Autodesk Fusion 360 part; units mm, degrees
sketch "Sketch1" plane through (0, 0, 0) normal (0, 0, 1) x (1, 0, 0)
  line L0 (0, 0) -> (-12.1, 6.9859) construction
  line L1 (0, 0) -> (0, -13.9719) construction
  line L2 (0, 0) -> (12.1, 6.9859) construction
  line L3 (12.1, -20.9578) -> (24.2, -13.9719)
  line L4 (24.2, -13.9719) -> (24.2, 0)
  line L5 (24.2, 0) -> (12.1, 6.9859)
  line L6 (12.1, 6.9859) -> (0, 0)
  line L7 (0, 0) -> (0, -13.9719)
  line L8 (0, -13.9719) -> (12.1, -20.9578)
  line L9 (12.1, 6.9859) -> (12.1, 20.9578)
  line L10 (12.1, 20.9578) -> (0, 27.9438)
  line L11 (0, 27.9438) -> (-12.1, 20.9578)
  line L12 (-12.1, 20.9578) -> (-12.1, 6.9859)
  line L13 (-12.1, 6.9859) -> (0, 0)
  line L14 (0, 0) -> (12.1, 6.9859) construction
  line L15 (0, -13.9719) -> (0, 0) construction
  line L16 (0, 0) -> (-12.1, 6.9859)
  line L17 (-12.1, 6.9859) -> (-24.2, 0)
  line L18 (-24.2, 0) -> (-24.2, -13.9719)
  line L19 (-24.2, -13.9719) -> (-12.1, -20.9578)
  line L20 (-12.1, -20.9578) -> (0, -13.9719)
  point P0 (12.1, -6.9859)
  point P1 (0, 13.9719)
  point P2 (-12.1, -6.9859)
  dimension "d3" = 120
  dimension "d4" = 120
  dimension "d5" = 12.1
  dimension "d6" = 12.1
  dimension "d7" = 12.1
extrude "Extrude1" add sketch "Sketch1" along normal blind 3
sketch "Sketch2" plane through (0, 0, 3) normal (0, 0, 1) x (1, 0, 0)
  line L0 (-12.1, -20.9578) -> (0, -13.9719)
  line L1 (0, -13.9719) -> (12.1, -20.9578)
  line L2 (12.1, -20.9578) -> (24.2, -13.9719)
  line L3 (24.2, -13.9719) -> (24.2, 0)
  line L4 (24.2, 0) -> (12.1, 6.9859)
  line L5 (12.1, 6.9859) -> (12.1, 20.9578)
  line L6 (12.1, 20.9578) -> (0, 27.9438)
  line L7 (0, 27.9438) -> (-12.1, 20.9578)
  line L8 (-12.1, 20.9578) -> (-12.1, 6.9859)
  line L9 (-12.1, 6.9859) -> (-24.2, 0)
  line L10 (-24.2, 0) -> (-24.2, -13.9719)
  line L11 (-24.2, -13.9719) -> (-12.1, -20.9578)
  line L12 (15, 1.1) -> (-15, 1.1)
  line L13 (-15, 1.1) -> (-15, 3.1)
  line L14 (-15, 3.1) -> (15, 3.1)
  line L15 (15, 3.1) -> (15, 1.1)
  line L16 (15, -1.1) -> (-15, -1.1)
  line L17 (-15, -1.1) -> (-15, -3.1)
  line L18 (-15, -3.1) -> (15, -3.1)
  line L19 (15, -3.1) -> (15, -1.1)
  line L20 (24.2, -13.9719) -> (-12.1, 6.9859) construction
  line L21 (-24.2, -13.9719) -> (12.1, 6.9859) construction
  line L22 (0, 27.9438) -> (0, -13.9719) construction
  line L23 (24.2, -13.9719) -> (24.2, 0)
  line L24 (24.2, 0) -> (-24.2, 0) construction
  dimension "d10" = 30
  dimension "d11" = 2
  dimension "d16" = 2.2
extrude "Extrude2" add sketch "Sketch2" along normal blind 7 contours L12 L13 L14 L15 | L16 L17 L18 L19
sketch "Sketch3" plane through (0, 0, 0) normal (0, 0, -1) x (-1, 0, 0)
  line L0 (0, -13.9719) -> (12.1, -20.9578)
  line L1 (12.1, -20.9578) -> (24.2, -13.9719)
  line L2 (24.2, -13.9719) -> (24.2, 0)
  line L3 (24.2, 0) -> (12.1, 6.9859)
  line L4 (12.1, 6.9859) -> (12.1, 20.9578)
  line L5 (12.1, 20.9578) -> (0, 27.9438)
  line L6 (0, 27.9438) -> (-12.1, 20.9578)
  line L7 (-12.1, 20.9578) -> (-12.1, 6.9859)
  line L8 (-12.1, 6.9859) -> (-24.2, 0)
  line L9 (-24.2, 0) -> (-24.2, -13.9719)
  line L10 (-24.2, -13.9719) -> (-12.1, -20.9578)
  line L11 (-12.1, -20.9578) -> (0, -13.9719)
  line L12 (-15, 1.05) -> (15, 1.05)
  line L13 (15, 1.05) -> (15, -1.05)
  line L14 (15, -1.05) -> (-15, -1.05)
  line L15 (-15, -1.05) -> (-15, 1.05)
  line L16 (-15, 0) -> (15, 0) construction
  line L17 (0, -1.05) -> (0, 1.05) construction
  dimension "d19" = 30
  dimension "d20" = 2.1
extrude "Extrude3" cut sketch "Sketch3" against normal blind 2 contours L12 L13 L14 L15
fillet "Fillet1" radius 4 4 edges at (15, 2.1, 10) (15, -2.1, 10) (-15, 2.1, 10) (-15, -2.1, 10)
fillet "Fillet2" radius 2 9 edges at (-12.1, -20.9578, 1.5) (12.1, -20.9578, 1.5) (24.2, -13.9719, 1.5) (24.2, 0, 1.5) (12.1, 20.9578, 1.5) (0, 27.9438, 1.5) (-12.1, 20.9578, 1.5) (-24.2, 0, 1.5) (-24.2, -13.9719, 1.5)
fillet "Fillet3" radius 0.5 4 edges at (0, -1.05, 0) (0, 1.05, 0) (-15, 0, 0) (15, 0, 0)
fillet "Fillet5" radius 2 21 edges at (12.1, 13.3945, 3) (11.8321, 20.8031, 3) (6.05, 24.4508, 3) (0, 27.6344, 3) (-6.05, 24.4508, 3) (-11.8321, 20.8031, 3) (-12.1, 13.3945, 3) (5.55, -17.1762, 3) (12.1, -20.6484, 3) (18.15, -17.4648, 3) (23.9321, -13.8172, 3) (24.2, -6.9859, 3) (23.9321, -0.1547, 3) (17.65, 3.7816, 3) (-17.65, 3.7816, 3) (-23.9321, -0.1547, 3) (-24.2, -6.9859, 3) (-23.9321, -13.8172, 3) (-18.15, -17.4648, 3) (-12.1, -20.6484, 3) (-5.55, -17.1762, 3)
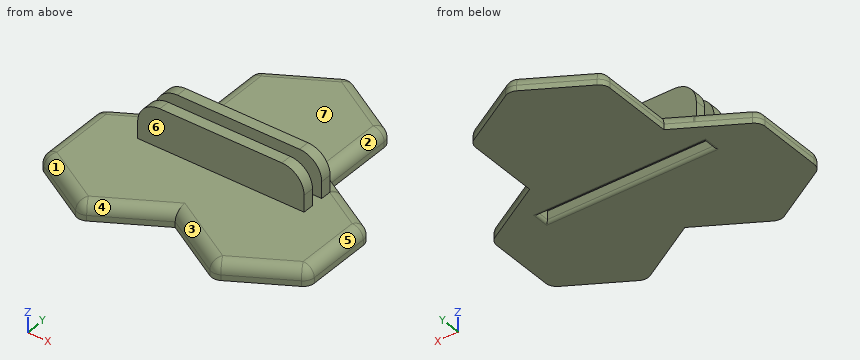
Verification items for the finished model (mm, model axes). Face numbers are marked on the shaded views. A direction names the side the tool comes from. Coordinates: 2 decimals unless noted, no trailing zeros. Order: outer loops, then holes, each group sorted by start corner. A loop starts at its lowest first (then second) coordinate and runs counter-clockwise, first axis right, second up. Notation, with made-up numbers: M -36.5,71 L -20.5,71 A25 cw -20.5,106 Z; hole C -18,-25 d8. An arc over 180 degrees is marked long. Return JSON: item names as keys, results as strings.
1) Release check for a two-part mould opening along X. For the marked faces 1, 2, 3 and 4 record: +X half, -X half, draft (parallel to the pull), parting line (faces both ways), or undercut.
Answer list:
{"face 1": "-X half", "face 2": "+X half", "face 3": "undercut", "face 4": "undercut"}
2) Cross-section at B-B, the plane y = 17.5. Record the boundary of the cut face in (x, z), and give its area (3 significant figures).
Answer list:
{"outline": "M -12.1,0 L 12.1,0 L 12.1,1 A2 ccw 10.1,3 L -10.1,3 A2 ccw -12.1,1 Z", "area": "70.9 mm2"}
3) Cross-section at C-C, the plane z = 7.5. Record the boundary of the cut face in (x, y), and give its area (3 significant figures).
Answer list:
{"outline": "M -14.71,-3.1 L 14.71,-3.1 L 14.71,-1.1 L -14.71,-1.1 Z; M -14.71,1.1 L 14.71,1.1 L 14.71,3.1 L -14.71,3.1 Z", "area": "118 mm2"}
4) Thickness scan on L1, parallel to Y at x = 14, z = 8.25; L2, parallel to Y at x = 0, z = 0.5; L3, parallel to Z at x = 1.5, y = 16.5. Record the ranges inside material, lowest first. Write a range as [from, to].
Answer list:
{"L1": "[-3.1, -1.1], [1.1, 3.1]", "L2": "[-13.97, -1.05], [1.05, 27.63]", "L3": "[0, 3]"}
5) Access from +Z, -Z, +X, -X, +Y, -Y to the whole of each face (thin tool, end or side, straight path). Record for the marked faces 5, 6 and 7.
Answer list:
{"face 5": "+Z, +X, +Y, -Y", "face 6": "+Z, +X, -X, -Y", "face 7": "+Z, +X, -X, +Y"}
6) Cross-section at D-D, the plane y = -8. Record the boundary of the cut face in (x, z), and give its area (3 significant figures).
Answer list:
{"outline": "M -24.2,0 L 24.2,0 L 24.2,1 A2 ccw 22.2,3 L -22.2,3 A2 ccw -24.2,1 Z", "area": "143 mm2"}
7) Cross-section at A-A, the plane z = 4.5. Record the boundary of the cut face in (x, y).
Answer list:
{"outline": "M -15,-3.1 L 15,-3.1 L 15,-1.1 L -15,-1.1 Z; M -15,1.1 L 15,1.1 L 15,3.1 L -15,3.1 Z"}
8) Gauge pin test, flat ends, axial feed: pin 1 (6 mm diameter, centred on x = 1.5, z = 7, fed in from +Y); pin 2 (5.5 mm diameter, centred on x = 3, z = 5, fed in from -Y); pin 3 (1 mm diameter, centred on x = -12, z = 2.5, fed in from -Y). Record the tip position at first contact, or that the pin passes through.
Answer list:
{"pin 1": "y = 3.1", "pin 2": "y = -15.58", "pin 3": "y = -20.38"}
